```python
from build123d import *

# Parameters (mm, degrees)
SKETCH2_R           = 60
BOSS_EXTRUDE2_DEPTH = 10
SKETCH3_R           = 2
CUT_EXTRUDE1_DEPTH  = 86.440037453


with BuildPart() as part:
    # Sketch2 → Boss-Extrude2 (new body)
    with BuildSketch(Plane(origin=(0, 0, 0), x_dir=(1, 0, 0), z_dir=(0, 1, 0))):
        with Locations(Location((0, 0, 0), (0, 0, 270))):
            Circle(SKETCH2_R)
        with BuildLine():
            Line((-8.979157617, -38.979157617), (-8.979157617, -8.979157617))
            Line((-8.979157617, -8.979157617), (-38.979157617, -8.979157617))
            ThreePointArc((-38.979157617, -8.979157617), (-28.284271247, -28.284271247), (-8.979157617, -38.979157617))
        make_face(mode=Mode.SUBTRACT)
        with BuildLine():
            Line((-8.979157617, 8.979157617), (-8.979157617, 38.979157617))
            ThreePointArc((-8.979157617, 38.979157617), (-28.284271247, 28.284271247), (-38.979157617, 8.979157617))
            Line((-38.979157617, 8.979157617), (-8.979157617, 8.979157617))
        make_face(mode=Mode.SUBTRACT)
        with BuildLine():
            Line((8.979157617, 8.979157617), (38.979157617, 8.979157617))
            ThreePointArc((38.979157617, 8.979157617), (28.284271247, 28.284271247), (8.979157617, 38.979157617))
            Line((8.979157617, 38.979157617), (8.979157617, 8.979157617))
        make_face(mode=Mode.SUBTRACT)
        with BuildLine():
            Line((8.979157617, -8.979157617), (8.979157617, -38.979157617))
            ThreePointArc((8.979157617, -38.979157617), (28.284271247, -28.284271247), (38.979157617, -8.979157617))
            Line((38.979157617, -8.979157617), (8.979157617, -8.979157617))
        make_face(mode=Mode.SUBTRACT)
    extrude(amount=BOSS_EXTRUDE2_DEPTH)

    # Sketch3 → Cut-Extrude1 (cut, through all)
    with BuildSketch(Plane.XZ):
        with Locations(Location((-10.5, 0, 0), (0, 0, 270))):
            Circle(SKETCH3_R)
        with Locations(Location((0, 10.5, 0), (0, 0, 270))):
            Circle(SKETCH3_R)
        with Locations(Location((10.5, 0, 0), (0, 0, 270))):
            Circle(SKETCH3_R)
        with Locations(Location((0, -10.5, 0), (0, 0, 270))):
            Circle(SKETCH3_R)
    extrude(amount=-CUT_EXTRUDE1_DEPTH, mode=Mode.SUBTRACT)


solid = part.part
```
Work out the finished part from the listing and answer in its coordinate system (mm). A direction names the side the tool comes from. Round coordinates to 2 decimals unless told otherwise and drop trailing zeros. Write each loop counter-clockwise with the first axis right and the second up, starting at its lowest first coordinate (ties: lowest second). Pieces come first, ordered by that corner, then holes.
1) Consider probe 1 along X at (y, z) = (5, 0); probe 2 along X at (y, z) = (4, 10.5); probe 3 along Z at (x, y) = (27, 3.5). Determine where each line is inside the solid, lowest interval first.
2) A cutting plane is placed at D-D on z = -41.5. Determine the outline of the cut face in (x, y), and give its area (3 significant figures).
3) A cutting plane is placed at B-B on y = 8.25. Give the number of separate pieces and of enclosed holes in the cut face, and give its area (3 significant figures).
4) Flat-ended cylindrical pins translate along their axes: P1, Ø4, axis at y = 3, z = -43, coming from the +X side; P2, Ø6, axis at x = 33.5, y = 5.5, coming from the -Z side; P3, Ø5, axis at y = 7.5, z = 23.5, coming from the +X side (3 decimals); P4, Ø2.5, axis at x = 0, z = 10.5, coming from the -Y side. Find the tip coordinate at first contact, or state that the pin passes through.
5) A cutting plane is placed at C-C on z = 0. Determine the outline of the cut face in (x, y).
6) Which of the six approach directions +Z, -Z, +X, -X, +Y, -Y give full straight-line access (tool end or side, diameter ignored) to faces 4 (the face through (24, 5, 8.979)), 5 (the face through (1, 10, -1))?
7) A cutting plane is placed at A-A on x = 0. Determine the outline of the cut face in (y, z).
8) Determine the mould class of faces 1 (the face through (24, 5, -8.979)), 2 (the face through (2.64, 4.93, -59.94)), 3 (the face through (1, 0, -1)) for opening direction Z: pulls with the +Z half, pulls with the -Z half, needs draft (parallel to the pull), parting line crosses it, or undercut.
Entries:
1. probe 1: x = -60 to -12.5, -8.5 to 8.5, 12.5 to 60
1. probe 2: x = -59.07 to -38.6, -8.98 to -2, 2 to 8.98, 38.6 to 59.07
1. probe 3: z = -53.58 to -29.51, -8.98 to 8.98, 29.51 to 53.58
2. outline: (-43.33, 0) - (43.33, 0) - (43.33, 10) - (-43.33, 10) - close
2. area: 867 mm2
3. separate pieces: 1
3. enclosed holes: 8
3. area: 8,760 mm2
4. P1: stops at x = 43.81
4. P2: stops at z = -51.67
4. P3: stops at x = 56.205
4. P4: passes through
5. outline: (-60, 0) - (-12.5, 0) - (-12.5, 10) - (-60, 10) - close; (-8.5, 0) - (8.5, 0) - (8.5, 10) - (-8.5, 10) - close; (12.5, 0) - (60, 0) - (60, 10) - (12.5, 10) - close
6. face 4: +Y, -Y
6. face 5: +Z, -Z, +X, -X, +Y
7. outline: (0, -60) - (10, -60) - (10, -12.5) - (0, -12.5) - close; (0, -8.5) - (10, -8.5) - (10, 8.5) - (0, 8.5) - close; (0, 12.5) - (10, 12.5) - (10, 60) - (0, 60) - close
8. face 1: undercut
8. face 2: parting line crosses it
8. face 3: needs draft
